Could you check a few things on this model? Use its own coordinates, in mm. A direction names the side the tool comes from. Round coordinates to 2 decimals unless told otherwise and drop trailing zeros. Write each loop counter-clockwise with the first axis right and the second up, starting at its lowest first coordinate (ties: lowest second). Pieces come first, ordered by that corner, then holes. Notation, with made-up numbers: M 30.25,10.25 L 88.25,10.25 A23 cw 88.25,25.25 Z; hole C -20,56 d10. An arc over 180 degrees is marked long. One line per item, written item: value. Start each with the question number.
(1) Which directions (+Z, -Z, +X, -X, +Y, -Y) give clear straight access to the entire face, cutting with the end or side of a thin tool? Please do faces 1 (the face through (-45, -11, 7)), 2 (the face through (0, -52, 7)), 3 (the face through (-12, -49.5, 7)), 4 (the face through (-43, -13, 7)).
(2) Thinking about a two-plate mould opening in Y: for faces 5 (the face through (45, 11, 7)), 6 (the face through (-1, 1, 0)), 7 (the face through (-41.3, -27.94, 1.52)), which applies, released by +Y, released by -Y, zero draft, split by the parting line, or undercut?
(3) If I drill on L1, parallel to X at y = 7, z = 6; L2, parallel to Y at x = -1, z = 2.25; L3, parallel to Z at x = -19.5, y = 8, over which ranges is the centre line in solid material (lowest first)?
(4) I want a section at A-A on z = 5. Please give me the cut outline in (x, y), and give its area (3 significant figures).
(5) I want a section at C-C on x = 40. Please give me the cut outline in (y, z).
(6) I'm going to push flat-ended pins straight in: pin 1 Ø4 at (y, z) = (34.5, 1.5) entering from +X; pin 2 Ø0.6 at (y, z) = (-12.5, 7) entering from -X; pin 3 Ø1.5 at (x, z) = (9, 8) entering from -Y; pin 4 Ø5 at (x, y) = (9, -7.5) entering from -Z. Where does each tip first touch, or does it pass through?
(7) I want a section at D-D on y = 3.5. Please give me the cut outline in (x, z).
(8) I want a section at B-B on y = 18. Please give me the cut outline in (x, z), and give its area (3 significant figures).
```python
from build123d import *

# Parameters (mm, degrees)
SKETCH_R     = 55
PAD_DEPTH    = 3
PAD001_DEPTH = 8
PAD002_DEPTH = 8
SKETCH003_R  = 1.3
POCKET_DEPTH = 5


with BuildPart() as part:
    # Sketch → Pad (new body)
    with BuildSketch(Plane.XY):
        Circle(SKETCH_R)
    extrude(amount=PAD_DEPTH)

    # Sketch001 (on Face3 of Pad) → Pad001 (join)
    with BuildSketch(Plane.XY.offset(3)):
        Polygon((33.500008, 0), (33.500008, 13), (53.345406, 13), (53.345406, 11), (35.5, 11), (35.5, -0.005684), (35.5, -12), (33.500008, -12), align=None)
        Polygon((-33.5, 0), (-33.5, -13), (-53.293575, -13), (-53.293575, -11), (-35.5, -11), (-35.5, 0.001212), (-35.5, 12), (-33.5, 12), align=None)
    extrude(amount=PAD001_DEPTH)

    # Sketch002 (on Face3 of Pad001) → Pad002 (join)
    with BuildSketch(Plane.XY.offset(3)):
        with BuildLine():
            ThreePointArc((-23.973944, -49.5), (-12.298374, -53.607369), (0, -55))
            Line((0, -49.5), (0, -55))
            Line((-23.973944, -49.5), (0, -49.5))
        make_face()
        with BuildLine():
            ThreePointArc((23.973944, 49.5), (12.298374, 53.607369), (0, 55))
            Line((0, 49.5), (0, 55))
            Line((23.973944, 49.5), (0, 49.5))
        make_face()
    extrude(amount=PAD002_DEPTH)

    # Sketch003 (on Face3 of Pad002) → Pocket (cut)
    with BuildSketch(Plane.XY.offset(3)):
        with Locations((-45, -18)):
            Circle(SKETCH003_R)
        with Locations((45, 18)):
            Circle(SKETCH003_R)
        with Locations((-40, -28)):
            Circle(SKETCH003_R)
        with Locations((40, 28)):
            Circle(SKETCH003_R)
    extrude(amount=-POCKET_DEPTH, mode=Mode.SUBTRACT)


solid = part.part
```
Found:
1. face 1: +Z, -X, +Y
1. face 2: +Z, +X, -Y
1. face 3: +Z, +X, -X, +Y
1. face 4: +Z, +X, -X, -Y
2. face 5: released by -Y
2. face 6: zero draft
2. face 7: undercut
3. L1: x = -35.5 to -33.5, 33.5 to 35.5
3. L2: y = -54.99 to 54.99
3. L3: z = 0 to 3
4. outline: M -53.29,-13 L -33.5,-13 L -33.5,12 L -35.5,12 L -35.5,-11 L -53.29,-11 Z; M -23.97,-49.5 A55 ccw 0,-55 L 0,-49.5 Z; M 0,49.5 L 23.97,49.5 A55 ccw 0,55 Z; M 33.5,-12 L 35.5,-12 L 35.5,11 L 53.35,11 L 53.35,13 L 33.5,13 Z
4. area: 349 mm²
5. outline: M -37.75,0 L 26.7,0 L 26.7,3 L 13,3 L 13,11 L 11,11 L 11,3 L -37.75,3 Z; M 29.3,0 L 37.75,0 L 37.75,3 L 29.3,3 Z
6. pin 1: stops at x = 44.37
6. pin 2: stops at x = -53.29
6. pin 3: stops at y = 49.5
6. pin 4: stops at z = 0
7. outline: M -54.89,0 L 54.89,0 L 54.89,3 L 35.5,3 L 35.5,11 L 33.5,11 L 33.5,3 L -33.5,3 L -33.5,11 L -35.5,11 L -35.5,3 L -54.89,3 Z
8. outline: M -51.97,0 L 43.7,0 L 43.7,3 L -51.97,3 Z; M 46.3,0 L 51.97,0 L 51.97,3 L 46.3,3 Z
8. area: 304 mm²
